from build123d import *

# Parameters (mm, degrees)
F0_W     = 101.6
F0_H     = 376.3636363636
F1_DEPTH = 50.8
F2_W     = 88.9
F2_H     = 88.9
F3_DEPTH = 1476.9896363636
F4_R     = 2.5


with BuildPart() as f1:
    # F0 (on Top) → F1 (new body, symmetric)
    with BuildSketch(Plane.XY):
        Polygon((560, -75), (560, 75), (458.4, -75), (458.4, -658.6363636364), (560, -658.6363636364), align=None)
        Polygon((458.4, -75), (560, 75), (560, 301.3636363636), (560, 451.3636363636), (458.4, 301.3636363636), align=None)
        with Locations((509.2, -846.8181818182)):
            Rectangle(F0_W, F0_H)
    extrude(amount=F1_DEPTH, both=True)

    # F2 (on face) → F3 (cut, through all)
    with BuildSketch(Plane.XZ.offset(1035)):
        with Locations((509.2, 0)):
            Rectangle(F2_W, F2_H)
    extrude(amount=-F3_DEPTH, mode=Mode.SUBTRACT)

    # F4
    f4_edges = [f1.edges().sort_by_distance(p)[0] for p in [
        (560, -291.818182, 50.8),
        (458.4, -366.818182, 50.8),
        (458.4, -366.818182, -50.8),
        (560, -291.818182, -50.8),
        (464.75, -362.130682, 44.45),
        (553.65, -296.505682, 44.45),
        (553.65, -296.505682, -44.45),
        (464.75, -362.130682, -44.45),
    ]]
    fillet(f4_edges, radius=F4_R)


solid = f1.part
Build history of the part. All positions in model axes, mm. A direction names the side the tool comes from. Coordinates: 2 decimals unless noted, no trailing zeros. Write each loop counter-clockwise with the first axis right and the second up, starting at its lowest first coordinate (ties: lowest second). Pieces come first, ordered by that corner, then holes. Notation, with made-up numbers: (34.25, -27.75) -> (71.25, -27.75) arc R26 cw to (71.25, -0.75) -> close; hole circle Ø11 at (23.25, 73.25). An arc over 180 degrees is marked (long way). Use CSV: the item, a comma, the result in double quotes. Start each with the question number.
Q1. Drill centre lines: probe 1 along X at (y, z) = (3.5, -37.5); probe 2 along Z at (x, y) = (473, -321); probe 3 along X at (y, z) = (-216.5, 44). Where is each one in solid material? Low to high.
Q2. Cut at B-B, the plane x = 483. List the corners of the cut face in (y, z).
Q3. 3-axis set-ups, long thin cutter, end or side, ignore diameter. For faces 1 (the flat face through (509, -309, -44.45)), 2 (the flat face through (464, -1035, 0)): which of +Z, -Z, +X, -X, +Y, -Y reach the whole face in a straight line?
Q4. Pull direction Z, two halves, no side cores. Call faces 3 (the flat face through (509, -283, 50.8)), 4 (the flat face through (464.75, -372, -1)), 5 (the flat face through (509.437, 376.714, 45.393)): released by +Z, released by -Z, zero draft, split by the parting line, or undercut.
Q5. Cut at C-C, the plane y = 199. List the corners of the cut face in (x, z).
Q6. Cut at A-A, the plane z = 8. List the corners of the cut face in (x, y).
Checked values:
1,probe 1,"x = 458.4 to 464.75, 553.65 to 560"
1,probe 2,"z = -50.8 to -44.45, 44.45 to 50.8"
1,probe 3,"x = 458.4 to 465.82, 552.58 to 560"
2,outline,"(-1035, -50.8) -> (337.68, -50.8) -> (337.68, -44.45) -> (-1035, -44.45) -> close; (-1035, 44.45) -> (337.68, 44.45) -> (337.68, 50.8) -> (-1035, 50.8) -> close"
3,face 1,"+Y, -Y"
3,face 2,"+Z, -Z, +X, -X, -Y"
4,face 3,"released by +Z"
4,face 4,"undercut"
4,face 5,"zero draft"
5,outline,"(458.4, -48.3) arc R2.5 ccw to (460.9, -50.8) -> (557.5, -50.8) arc R2.5 ccw to (560, -48.3) -> (560, 48.3) arc R2.5 ccw to (557.5, 50.8) -> (460.9, 50.8) arc R2.5 ccw to (458.4, 48.3) -> close; hole (464.75, -41.95) arc R2.5 ccw to (467.25, -44.45) -> (551.15, -44.45) arc R2.5 ccw to (553.65, -41.95) -> (553.65, 41.95) arc R2.5 ccw to (551.15, 44.45) -> (467.25, 44.45) arc R2.5 ccw to (464.75, 41.95) -> close"
6,outline,"(458.4, -1035) -> (464.75, -1035) -> (464.75, 310.74) -> (458.4, 301.36) -> close; (553.65, -1035) -> (560, -1035) -> (560, 451.36) -> (553.65, 441.99) -> close"
